Check sheet for the modelled part. Datum: model origin and axes. Units: mm. Face numbers are marked on the shaded views. A direction names the side the tool comes from. Give positions to 0.01 mm unless a question says otherwise; leave off trailing zeros. Order: outer loops, then holes, each group sorted by start corner. A loop starts at its lowest first (then second) coordinate and runs counter-clockwise, first axis right, second up. Notation, with made-up numbers: (14.5, -33) -> (60.5, -33) arc R29 cw to (60.5, -11) -> close; hole circle Ø5 at (-6, 7.5). An arc over 180 degrees is marked (long way). One line per question, with ' | ' between items.
```python
from build123d import *

# Parameters (mm, degrees)
SKETCH1_W           = 78
SKETCH1_H           = 25
BOSS_EXTRUDE1_DEPTH = 10
SKETCH2_W           = 68
SKETCH2_H           = 15
CUT_EXTRUDE2_DEPTH  = 10
SKETCH3_W           = 25
SKETCH3_H           = 5
BOSS_EXTRUDE2_DEPTH = 10
SKETCH4_W           = 25
SKETCH4_H           = 5
BOSS_EXTRUDE3_DEPTH = 10
SKETCH6_W           = 10
SKETCH6_H           = 5
BOSS_EXTRUDE4_DEPTH = 5
SKETCH9_R           = 1.75
CUT_EXTRUDE5_DEPTH  = 2
SKETCH10_R          = 1
CUT_EXTRUDE6_DEPTH  = 13
CUT_EXTRUDE7_DEPTH  = 1.5
SKETCH12_R          = 1
CUT_EXTRUDE8_DEPTH  = 10.5
SKETCH13_R          = 1
CUT_EXTRUDE9_DEPTH  = 15
SKETCH14_R          = 1.75
CUT_EXTRUDE11_DEPTH = 1.5


with BuildPart() as part:
    # Sketch1 → Boss-Extrude1 (new body)
    with BuildSketch(Plane(origin=(0, 0, 0), x_dir=(1, 0, 0), z_dir=(0, 1, 0))):
        Rectangle(SKETCH1_W, SKETCH1_H)
    extrude(amount=BOSS_EXTRUDE1_DEPTH)

    # Sketch2 → Cut-Extrude2 (cut)
    with BuildSketch(Plane(origin=(0, 10, 0), x_dir=(1, 0, 0), z_dir=(0, 1, 0))):
        Rectangle(SKETCH2_W, SKETCH2_H)
    extrude(amount=-CUT_EXTRUDE2_DEPTH, mode=Mode.SUBTRACT)

    # Sketch3 → Boss-Extrude2 (add)
    with BuildSketch(Plane.ZY.offset(39)):
        with Locations((0, 2.5)):
            Rectangle(SKETCH3_W, SKETCH3_H)
    extrude(amount=BOSS_EXTRUDE2_DEPTH)

    # Sketch4 → Boss-Extrude3 (add)
    with BuildSketch(Plane(origin=(39, 0, 0), x_dir=(0, 0, -1), z_dir=(1, 0, 0))):
        with Locations((0, 2.5)):
            Rectangle(SKETCH4_W, SKETCH4_H)
    extrude(amount=BOSS_EXTRUDE3_DEPTH)

    # Sketch6 → Boss-Extrude4 (add)
    with BuildSketch(Plane(origin=(0, 5, 0), x_dir=(1, 0, 0), z_dir=(0, 1, 0))):
        with Locations((44, 0)):
            Rectangle(SKETCH6_W, SKETCH6_H)
        with Locations((-44, 0)):
            Rectangle(SKETCH6_W, SKETCH6_H)
    extrude(amount=BOSS_EXTRUDE4_DEPTH)

    # Sketch9 → Cut-Extrude5 (cut)
    with BuildSketch(Plane.XZ):
        with Locations(Location((-44, 6.25, 0), (0, 0, 270))):
            Circle(SKETCH9_R)
        with Locations(Location((-44, -6.25, 0), (0, 0, 270))):
            Circle(SKETCH9_R)
        with Locations(Location((44, 6.25, 0), (0, 0, 270))):
            Circle(SKETCH9_R)
        with Locations(Location((44, -6.25, 0), (0, 0, 270))):
            Circle(SKETCH9_R)
    extrude(amount=-CUT_EXTRUDE5_DEPTH, mode=Mode.SUBTRACT)

    # Sketch10 → Cut-Extrude6 (cut)
    with BuildSketch(Plane.XZ.offset(-2)):
        with Locations(Location((-44, 6.25, 0), (0, 0, 270))):
            Circle(SKETCH10_R)
        with Locations(Location((-44, -6.25, 0), (0, 0, 270))):
            Circle(SKETCH10_R)
        with Locations(Location((44, 6.25, 0), (0, 0, 270))):
            Circle(SKETCH10_R)
        with Locations(Location((44, -6.25, 0), (0, 0, 270))):
            Circle(SKETCH10_R)
    extrude(amount=-CUT_EXTRUDE6_DEPTH, mode=Mode.SUBTRACT)

    # Sketch11 → Cut-Extrude7 (cut)
    with BuildSketch(Plane.XZ):
        with BuildLine():
            ThreePointArc((0, 11.75), (-1.75, 10), (0, 8.25))
            Line((0, 8.25), (0, 11.75))
        make_face()
        with BuildLine():
            Line((0, 11.75), (0, 8.25))
            ThreePointArc((0, 8.25), (1.237436867, 8.762563133), (1.75, 10))
            ThreePointArc((1.75, 10), (1.237436867, 11.237436867), (0, 11.75))
        make_face()
    extrude(amount=-CUT_EXTRUDE7_DEPTH, mode=Mode.SUBTRACT)

    # Sketch12 → Cut-Extrude8 (cut)
    with BuildSketch(Plane.XZ.offset(-1.5)):
        with Locations(Location((0, 10, 0), (0, 0, 270))):
            Circle(SKETCH12_R)
    extrude(amount=-CUT_EXTRUDE8_DEPTH, mode=Mode.SUBTRACT)

    # Sketch13 → Cut-Extrude9 (cut)
    with BuildSketch(Plane.XZ):
        with Locations(Location((0, -10, 0), (0, 0, 270))):
            Circle(SKETCH13_R)
    extrude(amount=-CUT_EXTRUDE9_DEPTH, mode=Mode.SUBTRACT)

    # Sketch14 → Cut-Extrude11 (cut)
    with BuildSketch(Plane.XZ):
        with Locations(Location((0, -10, 0), (0, 0, 270))):
            Circle(SKETCH14_R)
    extrude(amount=-CUT_EXTRUDE11_DEPTH, mode=Mode.SUBTRACT)


solid = part.part
```
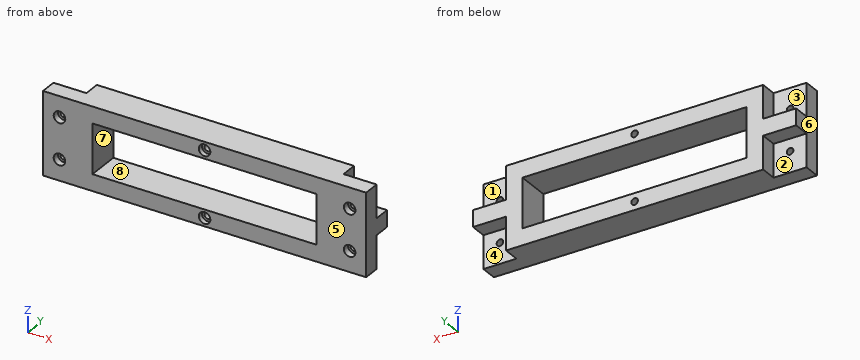
Q1. Section check A-A (z = -6.25). Enter the section's corners in (x, y), and give its area (3 significant figures).
Result sheet:
outline: (-49, 0) -> (-45.75, 0) -> (-45.75, 2) -> (-45, 2) -> (-45, 5) -> (-49, 5) -> close; (-43, 2) -> (-42.25, 2) -> (-42.25, 0) -> (-34, 0) -> (-34, 10) -> (-39, 10) -> (-39, 5) -> (-43, 5) -> close; (34, 0) -> (42.25, 0) -> (42.25, 2) -> (43, 2) -> (43, 5) -> (39, 5) -> (39, 10) -> (34, 10) -> close; (45, 2) -> (45.75, 2) -> (45.75, 0) -> (49, 0) -> (49, 5) -> (45, 5) -> close | area: 174 mm2
Q2. Depth check by flat-ended pin: pin 1 Ø1.5 at (y, z) = (6.5, -7) entering from -X; pin 2 Ø4 at (x, y) = (-41.5, 7.5) entering from +Z; pin 3 Ø3 at (x, z) = (44, -6.25) entering from -Y. Enter the tip coordinate at first touch or a pass-through.
Result sheet:
pin 1: stops at x = -39 | pin 2: stops at z = 2.5 | pin 3: stops at y = 2
Q3. Section check B-B (x = 23). Enter the section's corners in (y, z), and give its area (3 significant figures).
Result sheet:
outline: (0, -12.5) -> (10, -12.5) -> (10, -7.5) -> (0, -7.5) -> close; (0, 7.5) -> (10, 7.5) -> (10, 12.5) -> (0, 12.5) -> close | area: 100 mm2
Q4. Section check C-C (z = -10). Enter the section's corners in (x, y).
Result sheet:
outline: (-49, 0) -> (-1.75, 0) -> (-1.75, 1.5) -> (-1, 1.5) -> (-1, 10) -> (-39, 10) -> (-39, 5) -> (-49, 5) -> close; (1, 1.5) -> (1.75, 1.5) -> (1.75, 0) -> (49, 0) -> (49, 5) -> (39, 5) -> (39, 10) -> (1, 10) -> close
Q5. Mould release check, pull along X, two halves, no side actions. Record for the marked faces 5, 6, 7 and 8: pulls with the +X half, pulls with the -X half, needs draft (parallel to the pull), parting line crosses it, or undercut.
Result sheet:
face 5: needs draft | face 6: pulls with the -X half | face 7: undercut | face 8: undercut
Q6. Section check D-D (x = 44). Enter the section's corners in (y, z).
Result sheet:
outline: (0, -12.5) -> (5, -12.5) -> (5, -7.25) -> (2, -7.25) -> (2, -8) -> (0, -8) -> close; (0, -4.5) -> (2, -4.5) -> (2, -5.25) -> (5, -5.25) -> (5, -2.5) -> (10, -2.5) -> (10, 2.5) -> (5, 2.5) -> (5, 5.25) -> (2, 5.25) -> (2, 4.5) -> (0, 4.5) -> close; (0, 8) -> (2, 8) -> (2, 7.25) -> (5, 7.25) -> (5, 12.5) -> (0, 12.5) -> close
Q7. Access from +Z, -Z, +X, -X, +Y, -Y to the whole of each face (thin tool, end or side, straight path). Record for the marked faces 1, 2, 3 and 4.
Result sheet:
face 1: +Z, +X, +Y | face 2: -Z, -X, +Y | face 3: +Z, -X, +Y | face 4: -Z, +X, +Y
Q8. Thickness scan on line 1 (X direction, y = 2.75, z = -6.25); line 2 (X direction, y = 6.5, z = 0.5); line 3 (X direction, y = 8.75, z = 5.75). Record the ranges inside material, lowest first.
Result sheet:
line 1: x = -49 to -45, -43 to -34, 34 to 43, 45 to 49 | line 2: x = -49 to -34, 34 to 49 | line 3: x = -39 to -34, 34 to 39
